The listing builds one solid part. Answer for the finished solid, in the listing's coordinates (mm). A direction names the side the tool comes from. Give positions to 0.01 mm unless a question says otherwise; leave off trailing zeros. Loops run counter-clockwise (first coordinate to the right, second up) from the corner with the lowest first, then second, coordinate; pieces in that order, holes last. Notation, with made-up numbers: M 83,-15 L 91,-15 A14 ccw 91,2 Z; hole C 1.5,13 d9. An arc over 180 degrees is marked long. Return JSON: item names as keys, results as strings.
from build123d import *

# Parameters (mm, degrees)
SKETCH1_W                                         = 25.4
SKETCH1_H                                         = 19.05
SKETCH1_R                                         = 2.1463
SKETCH1_W_2                                       = 1.905
SKETCH1_H_2                                       = 6.35
BOSS_EXTRUDE1_DEPTH                               = 6.35
CSK_FOR_4_FLAT_HEAD_SOCKET_CAP_SCREW1_D           = 2.9464
CSK_FOR_4_FLAT_HEAD_SOCKET_CAP_SCREW1_CSINK_D     = 6.477
CSK_FOR_4_FLAT_HEAD_SOCKET_CAP_SCREW1_CSINK_ANGLE = 82
FILLET1_R                                         = 6.35


with BuildPart() as part:
    # Sketch1 → Boss-Extrude1 (new body)
    with BuildSketch(Plane(origin=(0, 0, 0), x_dir=(1, 0, 0), z_dir=(0, 1, 0))):
        with Locations((6.35, 0)):
            Rectangle(SKETCH1_W, SKETCH1_H)
        Circle(SKETCH1_R, mode=Mode.SUBTRACT)
        with Locations((5.3975, 0)):
            Rectangle(SKETCH1_W_2, SKETCH1_H_2, mode=Mode.SUBTRACT)
    extrude(amount=BOSS_EXTRUDE1_DEPTH)

    # CSK for #4 Flat Head Socket Cap Screw1 (through all)
    with Locations(Plane(origin=(0, 6.35, 0), x_dir=(1, 0, 0), z_dir=(0, 1, 0))):
        with Locations((2.54, 5.715), (15.24, -5.715), (2.54, -5.715), (15.24, 5.715)):
            CounterSinkHole(CSK_FOR_4_FLAT_HEAD_SOCKET_CAP_SCREW1_D / 2, CSK_FOR_4_FLAT_HEAD_SOCKET_CAP_SCREW1_CSINK_D / 2, counter_sink_angle=CSK_FOR_4_FLAT_HEAD_SOCKET_CAP_SCREW1_CSINK_ANGLE)

    # Fillet1
    fillet1_edges = [part.edges().sort_by_distance(p)[0] for p in [
        (-6.35, 3.175, -9.525),
        (-6.35, 3.175, 9.525),
    ]]
    fillet(fillet1_edges, radius=FILLET1_R)


solid = part.part
(1) The part is cut by section C-C (y = 3). Determine the outline of the cut face in (x, z) (3 decimals).
Values follow:
{"outline": "M -6.35,-3.175 A6.35 ccw 0,-9.525 L 19.05,-9.525 L 19.05,9.525 L 0,9.525 A6.35 ccw -6.35,3.175 Z; hole C 0,0 d4.293; hole C 2.54,-5.715 d2.946; hole C 2.54,5.715 d2.946; hole M 4.445,-3.175 L 6.35,-3.175 L 6.35,3.175 L 4.445,3.175 Z; hole C 15.24,-5.715 d2.946; hole C 15.24,5.715 d2.946"}
(2) Straight lines are drawn through the part: line 1 along Z through (x, y) = (2.54, 3.3) (3 decimals); line 2 along X through (y, z) = (3.75, -5.5); line 3 along X through (y, z) = (5, -1) (3 decimals). For each, find the intervals that lie inside material, in ascending order.
Values follow:
{"line 1": "-9.525 to -7.188, -4.242 to 4.242, 7.188 to 9.525", "line 2": "-5.91 to 1.08, 4 to 13.78, 16.7 to 19.05", "line 3": "-6.35 to -1.899, 1.899 to 4.445, 6.35 to 19.05"}
(3) A tool of negligible diameter and unlimited length cuts with its end or side. For faces 1 (the flat face through (6.35, 3, 0)), 2 (the flat face through (19.05, 3, 0)), from which of +Z, -Z, +X, -X, +Y, -Y can it reach the whole face along a straight path? Write none if from no direction.
Values follow:
{"face 1": "+Y, -Y", "face 2": "+Z, -Z, +X, +Y, -Y"}
(4) The part is cut by section B-B (z = 0). Determine the outline of the cut face in (x, y) (3 decimals), and give its area (3 significant figures).
Values follow:
{"outline": "M -6.35,0 L -2.146,0 L -2.146,6.35 L -6.35,6.35 Z; M 2.146,0 L 4.445,0 L 4.445,6.35 L 2.146,6.35 Z; M 6.35,0 L 19.05,0 L 19.05,6.35 L 6.35,6.35 Z", "area": "122 mm²"}
(5) The part is cut by section A-A (x = 2.54). Give the number of separate pieces and of enclosed holes in the cut face, and give its area (3 significant figures).
Values follow:
{"separate pieces": "3", "enclosed holes": "0", "area": "76.4 mm²"}
(6) Given pin 1 (1.8 mm diameter, centred on x = 15.24, z = 5.715, fed in from +Y); pin 2 (2 mm diameter, centred on x = -3.5, y = 5.5, fed in from +Z); pin 3 (3.5 mm diameter, centred on x = 15.24, z = -5.715, fed in from +Y), each flat-ended and moving along its own axis, determine where each tip first touches the part or whether it passes through.
Values follow:
{"pin 1": "through", "pin 2": "z = 9.01", "pin 3": "y = 4.64"}
